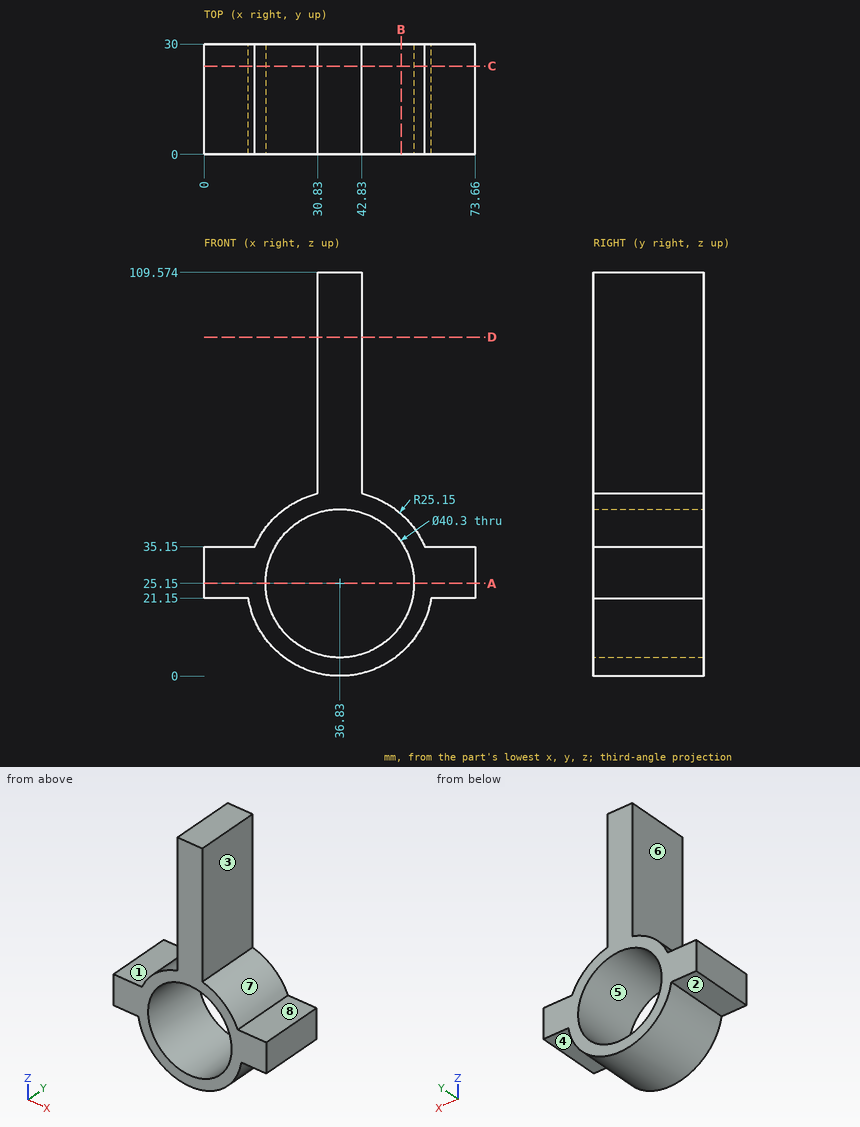
Answer from the drawing. Dimensions are ordinates in mm from the lowest x, y and z of the part. A direction names the side the tool comes from. Coordinates: 2 decimals unless noted, no trailing zeros. Loops run counter-clockwise (first coordinate to the right, second up) from the corner with the lowest first, then second, coordinate; pieces in that order, holes last. Notation, with made-up numbers: (14, -7.75) - (65, -7.75) arc R11 cw to (65, 0.25) - close; hole circle Ø10 at (23.25, -13.5). An arc over 180 degrees is marked (long way). Answer in a Markdown table with one row per item.
1. Straight lines are drawn through the part: line 1 (X direction, y = 10.75, z = 25.15); line 2 (X direction, y = 25, z = 64.5); line 3 (X direction, y = 2.25, z = 33). For each, find the intervals that lie inside material, in ascending order.
Conclusion:
| item | result |
|---|---|
| line 1 | x = 0 to 16.68, 56.98 to 73.66 |
| line 2 | x = 30.83 to 42.83 |
| line 3 | x = 0 to 18.27, 55.39 to 73.66 |
2. Find section A-A, the plane z = 25.15. Write down the section's boundary in (x, y), then the cut area to 3 significant figures.
Conclusion:
| item | result |
|---|---|
| outline | (0, 0) - (16.68, 0) - (16.68, 30) - (0, 30) - close; (56.98, 0) - (73.66, 0) - (73.66, 30) - (56.98, 30) - close |
| area | 1,000 mm² |
3. Find section C-C, the plane y = 24. Write down the section's boundary in (x, z), then the cut area to 3 significant figures.
Conclusion:
| item | result |
|---|---|
| outline | (0, 21.15) - (12, 21.15) arc R25.15 ccw to (61.66, 21.15) - (73.66, 21.15) - (73.66, 35.15) - (59.91, 35.15) arc R25.15 ccw to (42.83, 49.57) - (42.83, 109.57) - (30.83, 109.57) - (30.83, 49.57) arc R25.15 ccw to (13.75, 35.15) - (0, 35.15) - close; hole circle Ø40.3 at (36.83, 25.15) |
| area | 1,770 mm² |
4. Given pin 1 (3 mm diameter, centred on y = 8, z = 39.5, fed in from -X); pin 2 (5 mm diameter, centred on x = 21.5, y = 17.5, fed in from -Z); pin 3 (2 mm diameter, centred on y = 11.5, z = 77, fed in from +X), each flat-ended and moving along its own axis, determine where each tip first touches the part or whether it passes through.
Conclusion:
| item | result |
|---|---|
| pin 1 | stops at x = 15.21 |
| pin 2 | stops at z = 3.52 |
| pin 3 | stops at x = 42.83 |
5. Find section B-B, the plane x = 53.5. Write down the section's boundary in (y, z), then the cut area to 3 significant figures.
Conclusion:
| item | result |
|---|---|
| outline | (0, 6.32) - (30, 6.32) - (30, 13.83) - (0, 13.83) - close; (0, 36.47) - (30, 36.47) - (30, 43.98) - (0, 43.98) - close |
| area | 451 mm² |
6. Which of the six approach directions +Z, -Z, +X, -X, +Y, -Y give full straight-line access (tool end or side, diameter ignored) to the marked faces 1, 2, 3 and 4?
Conclusion:
| item | result |
|---|---|
| face 1 | +Z, -X, +Y, -Y |
| face 2 | -Z, -X, +Y, -Y |
| face 3 | +Z, +X, +Y, -Y |
| face 4 | -Z, +X, +Y, -Y |
7. Determine the mould class of the marked faces 5, 6, 7 and 8 for opening direction X: +X half, -X half, draft (parallel to the pull), parting line (faces both ways), or undercut.
Conclusion:
| item | result |
|---|---|
| face 5 | undercut |
| face 6 | -X half |
| face 7 | +X half |
| face 8 | draft |
8. Find section D-D, the plane z = 92. Write down the section's boundary in (x, y).
Conclusion:
| item | result |
|---|---|
| outline | (30.83, 0) - (42.83, 0) - (42.83, 30) - (30.83, 30) - close |
